Read the model definition and answer for the solid it produces. Units are mm, in the model's axes. Face numbers are marked on the shaded views. A direction names the side the tool comes from. Coordinates: 2 decimals unless noted, no trailing zeros. Write each loop counter-clockwise with the first axis right and the second up, starting at its lowest first coordinate (ties: lowest second). Pieces come first, ordered by that corner, then holes. Notation, with made-up numbers: (-37, -36) -> (-14, -36) arc R4 cw to (-14, -32) -> close; hole circle Ø10 at (37.25, 80). An arc over 180 degrees is marked (long way). Use CSV: the item, a comma, the result in double quotes.
Solid Edge part; units mm, degrees
sketch "Sketch1" plane through (0, 0, 0) normal (0, -1, 0) x (1, 0, 0)
  line L0 (-43.4817, 16.5287) -> (-43.4817, 41.5287)
  line L1 (-19.4817, 16.5287) -> (-19.4817, 41.5287)
  line L2 (-43.4817, 16.5287) -> (-19.4817, 16.5287)
  arc A0 (-19.4817, 41.5287) -> (-43.4817, 41.5287) centre (-31.4817, 41.5287) ccw
extrude "Protrusion1" add sketch "Sketch1" against normal blind 30
sketch "Sketch2" plane through (0, 0, 0) normal (0, -1, 0) x (1, 0, 0)
  circle A0 centre (-31.4817, 41.5287) radius 6
extrude "ExtrudedCutout_1" cut sketch "Sketch2" against normal blind 30
sketch "Sketch3" plane through (-43.4817, 15, 29.0287) normal (-1, 0, 0) x (0, -1, 0)
  line L0 (6, 12.5) -> (6, -2.5)
  line L1 (6, -2.5) -> (-6, -2.5)
  line L2 (-6, -2.5) -> (-6, 12.5)
  line L3 (-6, 12.5) -> (-6, 28.2339)
  line L4 (6, 28.2339) -> (-6, 28.2339)
  line L5 (6, 12.5) -> (6, 28.2339)
extrude "ExtrudedCutout_2" cut sketch "Sketch3" against normal blind 24
sketch "Sketch4" plane through (-31.4817, 15, 16.5287) normal (0, 0, -1) x (1, 0, 0)
  circle A0 centre (-98, 0) radius 25
extrude "ExtrudedProtrusion_2" add sketch "Sketch4" along normal blind 20
sketch "Sketch5" plane through (-31.4817, 15, 16.5287) normal (0, 0, -1) x (1, 0, 0)
  circle A0 centre (-98, 0) radius 25
extrude "ExtrudedProtrusion_3" add sketch "Sketch5" against normal blind 30
sketch "Sketch6" plane through (-31.4817, 15, 16.5287) normal (0, 0, -1) x (1, 0, 0)
  line L0 (-12, -15) -> (-95.0628, -24.8269)
  line L1 (-95.0628, 24.8269) -> (-95.0628, -24.8269)
  line L2 (-12, 15) -> (-95.0628, 24.8269)
  line L3 (-12, 15) -> (-12, -15)
extrude "Protrusion2" add sketch "Sketch6" against normal blind 10
sketch "Sketch7" plane through (-31.4817, 15, 16.5287) normal (0, 0, -1) x (1, 0, 0)
  circle A0 centre (-98, 0) radius 15
extrude "Cutout1" cut sketch "Sketch7" along normal mid plane 75.5501
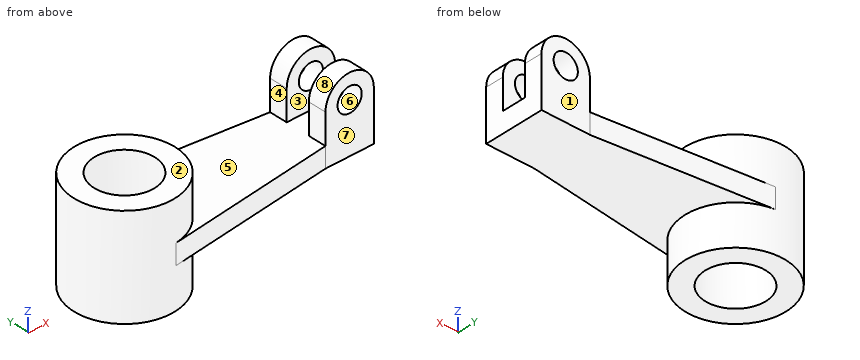
1. For a pull along Z with two mould halves and no side action, classify the marked faces 6, 7 and 8 as pulls with the +Z half, pulls with the -Z half, needs draft (parallel to the pull), parting line crosses it, or undercut.
Solutions:
face 6,"undercut"
face 7,"needs draft"
face 8,"pulls with the +Z half"
2. A cutting plane is placed at B-B (y = 3). Give the vertices of the cut face in (x, z).
Solutions:
outline,"(-151.41, -3.47) -> (-138.48, -3.47) -> (-138.48, 46.53) -> (-151.41, 46.53) -> close; (-120.48, -3.47) -> (-107.55, -3.47) -> (-107.55, 16.53) -> (-19.48, 16.53) -> (-19.48, 41.53) arc R12 ccw to (-43.48, 41.53) -> (-43.48, 26.53) -> (-107.55, 26.53) -> (-107.55, 46.53) -> (-120.48, 46.53) -> close; hole circle Ø12 at (-31.48, 41.53)"
3. A tool of negligible diameter and unlimited length cuts with its end or side. For the marked faces 1, 2, 3, 4 and 5, from which of +Z, -Z, +X, -X, +Y, -Y can it reach the whole face along a straight path? Write none if from no direction.
Solutions:
face 1,"+Z, -Z, +X, +Y"
face 2,"+Z, -X, +Y, -Y"
face 3,"+Z, +X"
face 4,"+Z, +Y, -Y"
face 5,"+Z"
4. A cutting plane is placed at C-C (z = 39.5). Give the vertices of the cut face in (x, y).
Solutions:
outline,"circle Ø50 at (-129.48, 15); (-43.48, 0) -> (-37.13, 0) -> (-37.13, 9) -> (-43.48, 9) -> close; (-43.48, 21) -> (-37.13, 21) -> (-37.13, 30) -> (-43.48, 30) -> close; (-25.84, 0) -> (-19.48, 0) -> (-19.48, 9) -> (-25.84, 9) -> close; (-25.84, 21) -> (-19.48, 21) -> (-19.48, 30) -> (-25.84, 30) -> close; hole circle Ø30 at (-129.48, 15)"
5. Each of these flat-tipped pins is pushed along its axis until it touches: pin 1 Ø19 at (x, z) = (-27.5, 45.5) entering from +Y; pin 2 Ø8 at (y, z) = (20, 14.5) entering from -X; pin 3 Ø10 at (y, z) = (27.5, 34) entering from -X. Where does it stop, or does it pass through?
Solutions:
pin 1,"stops at y = 30"
pin 2,"stops at x = -154.46"
pin 3,"stops at x = -153.33"
6. Find the intervals of material crossed by line 1 along Y through (x, z) = (-129, 0.5); line 2 along X through (y, z) = (4, 40.5); line 3 along Z through (x, y) = (-66, 18.5), in increasing order.
Solutions:
line 1,"y = -10 to 0.01, 29.99 to 40"
line 2,"x = -151.93 to -139.68, -119.28 to -107.03, -43.48 to -37.39, -25.57 to -19.48"
line 3,"z = 16.53 to 26.53"
7. A cutting plane is placed at A-A (z = 33.5). Give the vertices of the cut face in (x, y).
Solutions:
outline,"circle Ø50 at (-129.48, 15); (-43.48, 0) -> (-19.48, 0) -> (-19.48, 9) -> (-43.48, 9) -> close; (-43.48, 21) -> (-19.48, 21) -> (-19.48, 30) -> (-43.48, 30) -> close; hole circle Ø30 at (-129.48, 15)"
8. A cutting plane is placed at D-D (y = 15). Give the vertices of the cut face in (x, z).
Solutions:
outline,"(-154.48, -3.47) -> (-144.48, -3.47) -> (-144.48, 46.53) -> (-154.48, 46.53) -> close; (-114.48, -3.47) -> (-104.48, -3.47) -> (-104.48, 16.53) -> (-19.48, 16.53) -> (-19.48, 26.53) -> (-104.48, 26.53) -> (-104.48, 46.53) -> (-114.48, 46.53) -> close"
